```python
from build123d import *

# Parameters (mm, degrees)
SKETCH1_W            = 62
SKETCH1_H            = 38
SKETCH1_R            = 1.55
SKETCH1_W_2          = 40
SKETCH1_H_2          = 20
BOSS_EXTRUDE1_DEPTH  = 3
SKETCH3_W            = 86
SKETCH3_H            = 39
SKETCH3_W_2          = 62
SKETCH3_H_2          = 38
BOSS_EXTRUDE2_DEPTH  = 3
SKETCH4_R            = 1.75
CUT_EXTRUDE1_DEPTH   = 3
SKETCH5_R            = 2.55
CUT_EXTRUDE2_DEPTH   = 1.3
LPATTERN2_COUNT      = 4
LPATTERN2_PITCH      = 10
LPATTERN2_COUNT_DIR2 = 9
LPATTERN2_PITCH_DIR2 = 10


with BuildPart() as part:
    # Sketch1 → Boss-Extrude1 (new body)
    with BuildSketch(Plane.XY):
        Rectangle(SKETCH1_W, SKETCH1_H)
        with Locations((-27.873084587, 15.75)):
            Circle(SKETCH1_R, mode=Mode.SUBTRACT)
        with Locations((25.626915413, 15.75)):
            Circle(SKETCH1_R, mode=Mode.SUBTRACT)
        with Locations((-27.873084587, -14.55)):
            Circle(SKETCH1_R, mode=Mode.SUBTRACT)
        with Locations((25.626915413, -14.55)):
            Circle(SKETCH1_R, mode=Mode.SUBTRACT)
        Rectangle(SKETCH1_W_2, SKETCH1_H_2, mode=Mode.SUBTRACT)
    extrude(amount=BOSS_EXTRUDE1_DEPTH)

    # Sketch3 → Boss-Extrude2 (add)
    with BuildSketch(Plane.XY.offset(3)):
        Rectangle(SKETCH3_W, SKETCH3_H)
        Rectangle(SKETCH3_W_2, SKETCH3_H_2, mode=Mode.SUBTRACT)
    extrude(amount=-BOSS_EXTRUDE2_DEPTH)

    # Sketch4 → Cut-Extrude1 (cut)
    with BuildSketch(Plane(origin=(0, 0, 0), x_dir=(-1, 0, 0), z_dir=(0, 0, -1))):
        with Locations((-40, 16.5)):
            Circle(SKETCH4_R)
    cut_extrude1 = extrude(amount=-CUT_EXTRUDE1_DEPTH, mode=Mode.SUBTRACT)

    # Sketch5 → Cut-Extrude2 (cut)
    with BuildSketch(Plane.XY.offset(3)):
        with Locations((-27.873084587, 15.75)):
            Circle(SKETCH5_R)
        with Locations((-27.873084587, -14.55)):
            Circle(SKETCH5_R)
        with Locations((25.626915413, -14.55)):
            Circle(SKETCH5_R)
        with Locations((25.626915413, 15.75)):
            Circle(SKETCH5_R)
    extrude(amount=-CUT_EXTRUDE2_DEPTH, mode=Mode.SUBTRACT)

    # LPattern2: Cut-Extrude1 4 × 9, 28 skipped
    with Locations(*[(-j * LPATTERN2_PITCH_DIR2, -i * LPATTERN2_PITCH, 0) for i in range(LPATTERN2_COUNT) for j in range(LPATTERN2_COUNT_DIR2) if (i, j) not in ((0, 0), (0, 1), (0, 2), (0, 3), (0, 4), (0, 5), (0, 6), (0, 7), (1, 1), (1, 2), (1, 3), (1, 4), (1, 5), (1, 6), (1, 7), (2, 1), (2, 2), (2, 3), (2, 4), (2, 5), (2, 6), (2, 7), (3, 1), (3, 2), (3, 3), (3, 4), (3, 5), (3, 6), (3, 7))]):
        add(cut_extrude1, mode=Mode.SUBTRACT)


solid = part.part
```
Verification items for the finished model (mm, model axes). A direction names the side the tool comes from. Round coordinates to 2 decimals unless told otherwise and drop trailing zeros. Write each loop counter-clockwise with the first axis right and the second up, starting at its lowest first coordinate (ties: lowest second). Pieces come first, ordered by that corner, then holes.
1. Gauge pin test, flat ends, axial feed: P1, Ø3, axis at x = -40, y = -3.5, coming from the -Z side; P2, Ø1.5, axis at x = -28, y = -13.5, coming from the +Z side. Record the tip position at first contact, or that the pin passes through.
2. Section check A-A on y = 1. Enter the section's corners in (x, z).
3. Section check C-C on y = -3.5. Enter the section's corners in (x, z).
4. Scan lines: L1, parallel to Y at x = -40, z = 1.55; L2, parallel to X at y = -6, z = 2.75; L3, parallel to X at y = 8, z = 1.95. Record each from-to range of solid material in increasing order.
5. Section check D-D on z = 1.05. State how many separate pieces and enclosed holes the cut face has, plus the area to 3 significant figures.
6. Draft check along Y on faces 1 (the flat face through (-26, 16, 1.7)), 2 (the flat face through (-43, 0, 2)), 3 (the flat face through (27, -16, 1.7)), 4 (the flat face through (-1, 19.5, 2)). Enter one of: +Y half, -Y half, draft (parallel to the pull), parting line (faces both ways), or undercut.
7. Access from +Z, -Z, +X, -X, +Y, -Y to the whole of each face (thin tool, end or side, straight path). Record for faces 5 (the flat face through (43, 0, 2)), 6 (the cylindrical face through (23.6, 14.2, 2.4)), 7 (the flat face through (0, 10, 1)).
8. Section check B-B on x = -2. Enter the section's corners in (y, z), plus the area to 3 significant figures.
Answer:
1. P1: passes through
1. P2: stops at z = 1.7
2. outline: (-43, 0) - (-20, 0) - (-20, 3) - (-43, 3) - close; (20, 0) - (43, 0) - (43, 3) - (20, 3) - close
3. outline: (-43, 0) - (-41.75, 0) - (-41.75, 3) - (-43, 3) - close; (-38.25, 0) - (-20, 0) - (-20, 3) - (-38.25, 3) - close; (20, 0) - (38.25, 0) - (38.25, 3) - (20, 3) - close; (41.75, 0) - (43, 0) - (43, 3) - (41.75, 3) - close
4. L1: y = -19.5 to -15.25, -11.75 to -5.25, -1.75 to 4.75, 8.25 to 14.75, 18.25 to 19.5
4. L2: x = -43 to -20, 20 to 43
4. L3: x = -43 to -40.9, -39.1 to -20, 20 to 39.1, 40.9 to 43
5. separate pieces: 1
5. enclosed holes: 13
5. area: 2,450 mm2
6. face 1: undercut
6. face 2: draft
6. face 3: undercut
6. face 4: +Y half
7. face 5: +Z, -Z, +X, +Y, -Y
7. face 6: +Z
7. face 7: +Z, -Z
8. outline: (-19.5, 0) - (-10, 0) - (-10, 3) - (-19.5, 3) - close; (10, 0) - (19.5, 0) - (19.5, 3) - (10, 3) - close
8. area: 57.0 mm2
